The model under review builds one solid part; all positions refer to its coordinate system, in mm. Face numbers are marked on the shaded views. A direction names the side the tool comes from. Coordinates: 2 decimals unless noted, no trailing zeros. Order: outer loops, then holes, each group sorted by start corner. A loop starts at its lowest first (then second) coordinate and runs counter-clockwise, first axis right, second up. Notation, with made-up numbers: (39, -26) - (88, -26) arc R30 cw to (88, 2) - close; hole circle Ø8 at (82.25, 88). An arc over 180 degrees is marked (long way). Answer in a Markdown table with one row per item.
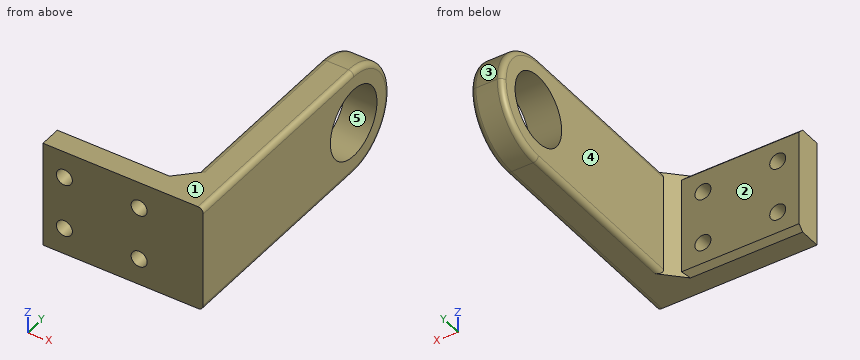
```python
from build123d import *

# Parameters (mm, degrees)
SKETCH1_W            = 150
SKETCH1_H            = 20
BOSS_EXTRUDE1_DEPTH  = 5
SKETCH2_W            = 20
SKETCH2_H            = 47
SKETCH2_R            = 6.5
BOSS_EXTRUDE2_DEPTH  = 6
FILLET1_R            = 10
FILLET1_OF_MIRROR1_R = 10
CHAMFER1_SIZE        = 2
FILLET2_R            = 1
CHAMFER2_SIZE        = 1
SKETCH3_W            = 35.580310247
SKETCH3_H            = 66.117820845
CUT_EXTRUDE1_DEPTH   = 120
SKETCH4_R            = 1.5
CUT_EXTRUDE2_DEPTH   = 10


with BuildPart() as part:
    # Sketch1 → Boss-Extrude1 (new body)
    with BuildSketch(Plane(origin=(0, 0, 0), x_dir=(1, 0, 0), z_dir=(0, 1, 0))):
        Rectangle(SKETCH1_W, SKETCH1_H)
    extrude(amount=BOSS_EXTRUDE1_DEPTH)

    # Sketch2 → Boss-Extrude2 (add)
    with BuildSketch(Plane.ZY.offset(75)):
        with Locations((0, 28.5)):
            Rectangle(SKETCH2_W, SKETCH2_H)
        with Locations((0, 42)):
            Circle(SKETCH2_R, mode=Mode.SUBTRACT)
    boss_extrude2 = extrude(amount=-BOSS_EXTRUDE2_DEPTH)

    # Fillet1
    fillet1_edges = [part.edges().sort_by_distance(p)[0] for p in [
        (-72, 52, -10),
        (-72, 52, 10),
    ]]
    fillet(fillet1_edges, radius=FILLET1_R - 0.0001)  # a hair under: the kernel refuses the full size

    # Mirror1: Boss-Extrude2 across plane
    add(boss_extrude2.mirror(Plane(origin=(0, 0, 0), x_dir=(0, 0, 1), z_dir=(1, 0, 0))))

    # Fillet1 of Mirror1
    fillet1_of_mirror1_edges = [part.edges().sort_by_distance(p)[0] for p in [
        (72, 52, -10),
        (72, 52, 10),
    ]]
    fillet(fillet1_of_mirror1_edges, radius=FILLET1_OF_MIRROR1_R - 0.0001)  # a hair under: the kernel refuses the full size

    # Chamfer1
    chamfer1_edges = [part.edges().sort_by_distance(p)[0] for p in [
        (-69, 5, 0),
        (69, 5, 0),
    ]]
    chamfer(chamfer1_edges, length=CHAMFER1_SIZE)

    # Fillet2
    fillet2_edges = [part.edges().sort_by_distance(p)[0] for p in [
        (-75, 21.00005, 10),
        (-75, 21.00005, -10),
        (-75, 49.071097101, 7.071097101),
        (-75, 49.071097101, -7.071097101),
        (-69, 24.50005, -10),
        (-69, 49.071097101, 7.071097101),
        (-69, 49.071097101, -7.071097101),
        (69, 24.50005, -10),
        (75, 21.00005, -10),
        (75, 21.00005, 10),
        (75, 49.071097101, 7.071097101),
        (75, 49.071097101, -7.071097101),
        (69, 49.071097101, 7.071097101),
        (69, 49.071097101, -7.071097101),
        (-69, 24.50005, 10),
        (69, 24.50005, 10),
    ]]
    fillet(fillet2_edges, radius=FILLET2_R)

    # Chamfer2
    chamfer2_edges = [part.edges().sort_by_distance(p)[0] for p in [
        (0, 5, -10),
        (0, 5, 10),
    ]]
    chamfer(chamfer2_edges, length=CHAMFER2_SIZE)

    # Sketch3 → Cut-Extrude1 (cut)
    with BuildSketch(Plane.ZY.offset(75)):
        with Locations((0.077756878, 33.058910422)):
            Rectangle(SKETCH3_W, SKETCH3_H)
    extrude(amount=-CUT_EXTRUDE1_DEPTH, mode=Mode.SUBTRACT)

    # Sketch4 → Cut-Extrude2 (cut)
    with BuildSketch(Plane(origin=(0, 5, 0), x_dir=(1, 0, 0), z_dir=(0, 1, 0))):
        with Locations(Location((49, 5, 0), (0, 0, 270))):
            Circle(SKETCH4_R)
        with Locations(Location((49, -5, 0), (0, 0, 270))):
            Circle(SKETCH4_R)
        with Locations(Location((63, -5, 0), (0, 0, 270))):
            Circle(SKETCH4_R)
        with Locations(Location((63, 5, 0), (0, 0, 270))):
            Circle(SKETCH4_R)
    extrude(amount=-CUT_EXTRUDE2_DEPTH, mode=Mode.SUBTRACT)


solid = part.part
```
Item 1: We need section A-A, the plane x = 49. Write out the cut boundary in (y, z), then the cut area to 3 significant figures.
Check values:
| item | result |
|---|---|
| outline | (0, -10) - (4, -10) - (5, -9) - (5, -6.5) - (0, -6.5) - close; (0, -3.5) - (5, -3.5) - (5, 3.5) - (0, 3.5) - close; (0, 6.5) - (5, 6.5) - (5, 9) - (4, 10) - (0, 10) - close |
| area | 69.0 mm^2 |
Item 2: We need section D-D, the plane y = 26. Write out the cut boundary in (x, z).
Check values:
| item | result |
|---|---|
| outline | (69, -9) arc R1 ccw to (70, -10) - (74, -10) arc R1 ccw to (75, -9) - (75, 9) arc R1 ccw to (74, 10) - (70, 10) arc R1 ccw to (69, 9) - close |
Item 3: We need section C-C, the plane x = 58.5. Write out the cut boundary in (y, z).
Check values:
| item | result |
|---|---|
| outline | (0, -10) - (4, -10) - (5, -9) - (5, 9) - (4, 10) - (0, 10) - close |
Item 4: Tool access review of the marked faces 1 and 2: name each direction out of +Z, -Z, +X, -X, +Y, -Y from which nothing blocks a thin tool from reaching the whole face with its end or side.
Check values:
| item | result |
|---|---|
| face 1 | +Z, +X, -X, +Y, -Y |
| face 2 | +Z, -Z, -X, +Y |
Item 5: Mouldability with a two-part tool opening along Z and no side actions: class the marked faces 3, 4 and 5 as +Z half, -Z half, draft (parallel to the pull), parting line (faces both ways), or undercut.
Check values:
| item | result |
|---|---|
| face 3 | +Z half |
| face 4 | draft |
| face 5 | undercut |
Item 6: We need section B-B, the plane y = 38.5. Write out the cut boundary in (x, z), then the cut area to 3 significant figures.
Check values:
| item | result |
|---|---|
| outline | (69, -9) arc R1 ccw to (70, -10) - (74, -10) arc R1 ccw to (75, -9) - (75, -5.48) - (69, -5.48) - close; (69, 5.48) - (75, 5.48) - (75, 9) arc R1 ccw to (74, 10) - (70, 10) arc R1 ccw to (69, 9) - close |
| area | 53.4 mm^2 |
Item 7: Clearance check with flat-ended pins moving along their axes: pin 1 Ø4 at (x, z) = (49, 5) entering from +Y; pin 2 Ø12 at (x, y) = (61.5, 18.5) entering from +Z. State where each tip first meets the part, or that it passes through.
Check values:
| item | result |
|---|---|
| pin 1 | y = 5 |
| pin 2 | through |
Item 8: To check wall thickness, follow line 1 (X direction, y = 2.6, z = 5); line 2 (X direction, y = 21, z = 4.5); line 3 (Y direction, x = 51.5, z = -4.5). State the ranges of each line that lie inside material, in increasing order. Write a range as from..to.
Check values:
| item | result |
|---|---|
| line 1 | 45..47.5, 50.5..61.5, 64.5..75 |
| line 2 | 69..75 |
| line 3 | 0..5 |
